Geometry: final body of the model. Coordinates: model frame, mm. A direction names the side the tool comes from. Coordinates: 2 decimals unless noted, no trailing zeros. Write each loop counter-clockwise with the first axis right and the second up, starting at its lowest first coordinate (ties: lowest second). Pieces come first, ordered by that corner, then holes. Notation, with made-up numbers: (-33, -7) -> (-6, -7) arc R9 cw to (-6, -1) -> close; hole circle Ø8 at (-7, -10). An arc over 180 degrees is marked (long way). Answer as a JSON object with one key per item and string values. Group by question number.
Autodesk Inventor part; units mm, degrees
ref_plane "YZ Plane" through (0, 0, 0) normal (1, 0, 0) x (0, 1, 0)
ref_plane "XZ Plane" through (0, 0, 0) normal (0, 1, 0) x (-1, 0, 0)
ref_plane "XY Plane" through (0, 0, 0) normal (0, 0, 1) x (1, 0, 0)
sketch "Sketch1" plane through (0, 0, 0) normal (0, 0, 1) x (1, 0, 0)
  line L0 (0, 0) -> (1.8311, 0)
  line L1 (0, 0) -> (0, 45.085)
  line L2 (0.381, 45.085) -> (0.381, 0.381)
  line L3 (0.381, 0.381) -> (1.8311, 0.381)
  line L4 (1.8311, 0.381) -> (1.8311, 0)
  line L5 (0.381, 45.085) -> (0, 45.085)
  dimension "d0" = 1.8311
  dimension "d1" = 45.085
  dimension "d2" = 0.381
extrude "Extrusion1" add sketch "Sketch1" along normal blind 88.9
fillet "Fillet1" radius 2.54 2 edges at (0.1905, 45.085, 88.9) (0.1905, 45.085, 0)
sketch "Sketch2" plane through (0, 0, 0) normal (-1, 0, 0) x (0, 0, 1)
  line L0 (0, 0) -> (88.9, 0)
  circle A0 centre (40.005, 0) radius 3.175
  circle A1 centre (48.895, 0) radius 3.2307
  dimension "d6" = 6.35
  dimension "d7" = 8.89
  dimension "d8" = 40.005
extrude "Extrusion2" cut sketch "Sketch2" against normal blind 88.9
sketch "Sketch3" plane through (0, 0, 0) normal (-1, 0, 0) x (0, 0, 1)
  circle A0 centre (20.1258, 30.6113) radius 3.175
  circle A1 centre (68.8299, 30.6113) radius 3.175
  line L0 (88.9, 42.545) -> (88.9, 0)
  line L1 (0, 42.545) -> (0, 0)
  line L2 (2.54, 45.085) -> (86.36, 45.085)
  line L3 (68.8299, 30.6113) -> (48.9507, 0)
  line L4 (48.9507, 0) -> (88.9, 0)
  line L5 (20.1258, 30.6113) -> (40.005, 0)
  line L6 (0, 0.381) -> (36.8529, 0.381)
  line L7 (40.005, 0) -> (0, 0)
  point P0 (52.1257, 0)
  point P1 (36.83, 0)
  dimension "d11" = 6.35
  dimension "d12" = 6.35
  dimension "d19" = 3.175
  dimension "d20" = 3.175
  dimension "d21" = 36.4998
  dimension "d22" = 45.085
  dimension "d23" = 45.085
  dimension "d24" = 36.4998
  dimension "d25" = 57
  dimension "d26" = 57
extrude "Extrusion3" cut sketch "Sketch3" against normal blind 88.9
sketch "Sketch4" plane through (0, 0, 88.9) normal (0, 0, 1) x (1, 0, 0)
  line L0 (-18.865, 53.0436) -> (15.9708, 53.0436)
  line L1 (15.9708, 53.0436) -> (15.9708, -6.5967)
  line L2 (15.9708, -6.5967) -> (-18.865, -6.5967)
  line L3 (-18.865, -6.5967) -> (-18.865, 53.0436)
  point P0 (0, 0)
extrude "Extrusion4" cut sketch "Sketch4" against normal blind 10.16
sketch "Sketch5" plane through (0, 0, 0) normal (0, 0, -1) x (-1, 0, 0)
  line L0 (-43.1556, 80.8845) -> (23.5088, 80.8845)
  line L1 (23.5088, 80.8845) -> (23.5088, -34.0438)
  line L2 (23.5088, -34.0438) -> (-43.1556, -34.0438)
  line L3 (-43.1556, -34.0438) -> (-43.1556, 80.8845)
  point P0 (0, 0)
extrude "Extrusion5" cut sketch "Sketch5" against normal blind 10.16
properties part number "Fin_short" material "Aluminum 6061"
Item 1: Mould query, pull axis Y, two halves, no side actions, for faces 1 (the flat face through (0.381, 23, 44)), 2 (the flat face through (1, 0.381, 65)), 3 (the cylindrical face through (0.188, 28.679, 17.606)). Classes: +Y half, -Y half, draft (parallel to the pull), parting line (faces both ways), or undercut.
Item 2: Ray query, L1, parallel to Y at x = 0.7, z = 24; L2, parallel to Z at x = 0.15, y = 32. Return the intervals inside material, ascending. Write a range as [from, to].
Item 3: Section B-B on z = 19. Output: boundary loops of the cut face in (x, y) (3 decimals).
Item 4: Set-up query: faces 4 (the flat face through (1, 0, 65)), 5 (the flat face through (1, 0.381, 23)). Return all of +Z, -Z, +X, -X, +Y, -Y with unobstructed straight access to the full face (end or side cutting, diameter ignored); none if empty.
Item 5: Section C-C on z = 27. Output: boundary loops of the cut face in (x, y) (3 decimals), then the cut area to 3 significant figures.
Item 6: Section A-A on x = 1.2. Output: boundary loops of the cut face in (y, z) (3 decimals), then the cut area to 3 significant figures.
Item 7: Section D-D on y = 11. Output: boundary loops of the cut face in (x, z).
Item 8: Contact query for flat-ended pins moving along their axis: pin 1 (4 mm diameter, centred on y = 9, z = 27, fed in from +X); pin 2 (8 mm diameter, centred on y = 28.5, z = 48.5, fed in from -X); pin 3 (1 mm diameter, centred on x = 1, y = 9.5, fed in from +Z). Output: stop coordinate, or through.
Answer sheet:
{
 "1": {"face 1": "draft", "face 2": "+Y half", "face 3": "undercut"},
 "2": {"L1": "y = [0, 0.38]", "L2": "z = [10.16, 17.27], [22.98, 65.97], [71.69, 78.74]"},
 "3": {"outline": "(0, 0) -> (1.831, 0) -> (1.831, 0.381) -> (0.381, 0.381) -> (0.381, 27.643) -> (0, 27.643) -> close; (0, 33.58) -> (0.381, 33.58) -> (0.381, 45.085) -> (0, 45.085) -> close"},
 "4": {"face 4": "+Z, -Z, +X, -X, -Y", "face 5": "+Z, -Z, +X, +Y"},
 "5": {"outline": "(0, 0) -> (1.831, 0) -> (1.831, 0.381) -> (0.381, 0.381) -> (0.381, 45.085) -> (0, 45.085) -> close", "area": "17.7 mm^2"},
 "6": {"outline": "(0, 10.16) -> (0.381, 10.16) -> (0.381, 36.853) arc R3.175 cw to (0, 36.83) -> close; (0, 43.18) arc R3.175 cw to (0.381, 43.157) -> (0.381, 45.687) arc R3.231 cw to (0, 45.664) -> close; (0, 52.126) arc R3.231 cw to (0.381, 52.103) -> (0.381, 78.74) -> (0, 78.74) -> close", "area": "21.3 mm^2"},
 "7": {"outline": "(0, 10.16) -> (0.38, 10.16) -> (0.38, 78.74) -> (0, 78.74) -> close"},
 "8": {"pin 1": "stops at x = 0.38", "pin 2": "stops at x = 0", "pin 3": "passes through"}
}
